CAD build for the part. Positions are in the model's coordinates, mm. Give positions to 0.01 mm unless a question says otherwise; leave off trailing zeros. Write each loop counter-clockwise with the first axis right and the second up, starting at its lowest first coordinate (ties: lowest second). Pieces come first, ordered by that corner, then holes. Notation, with made-up numbers: (-7.75, 39.25) -> (34.25, 39.25) arc R16 cw to (34.25, 65.25) -> close; hole circle Ø7 at (21.25, 83.25). An arc over 180 degrees is marked (long way). Answer in a Markdown table with one row per item. Add a question column.
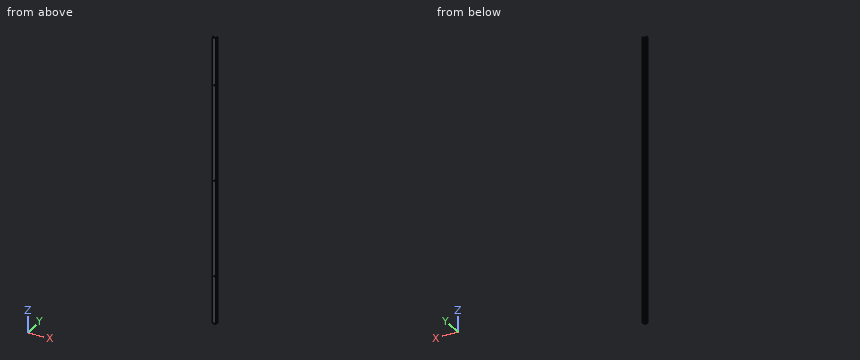
```python
from build123d import *

# Parameters (mm, degrees)
EXTRUDE_THIN1_DEPTH = 2997
SKETCH2_R           = 3.25
CUT_EXTRUDE1_DEPTH  = 2998.203367213
LPATTERN1_COUNT     = 3
LPATTERN1_PITCH     = 1000


with BuildPart() as part:
    # Sketch1 → Extrude-Thin1 (new body)
    with BuildSketch(Plane.XY):
        with BuildLine():
            Line((11.267326733, 18.158415842), (11.267326733, -6.841584158))
            ThreePointArc((11.267326733, -6.841584158), (10.388647076, -8.962904502), (8.267326733, -9.841584158))
            Line((8.267326733, -9.841584158), (-19.732673267, -9.841584158))
            ThreePointArc((-19.732673267, -9.841584158), (-21.853993611, -8.962904502), (-22.732673267, -6.841584158))
            Line((-22.732673267, -6.841584158), (-22.732673267, 18.158415842))
            Line((-22.732673267, 18.158415842), (-21.232673267, 18.158415842))
            Line((-21.232673267, 18.158415842), (-21.232673267, -6.841584158))
            ThreePointArc((-21.232673267, -6.841584158), (-20.793333439, -7.90224433), (-19.732673267, -8.341584158))
            Line((-19.732673267, -8.341584158), (8.267326733, -8.341584158))
            ThreePointArc((8.267326733, -8.341584158), (9.327986904, -7.90224433), (9.767326733, -6.841584158))
            Line((9.767326733, -6.841584158), (9.767326733, 18.158415842))
            Line((9.767326733, 18.158415842), (11.267326733, 18.158415842))
        make_face()
    extrude(amount=EXTRUDE_THIN1_DEPTH)

    # Sketch2 → Cut-Extrude1 (cut, through all)
    with BuildSketch(Plane(origin=(0, -8.341584158, 0), x_dir=(1, 0, 0), z_dir=(0, 1, 0))):
        with Locations(Location((-5.732673267, -2498.5, 0), (0, 0, 180))):
            Circle(SKETCH2_R)
    cut_extrude1 = extrude(amount=-CUT_EXTRUDE1_DEPTH, mode=Mode.SUBTRACT)

    # LPattern1: Cut-Extrude1 ×3
    with Locations(*[(0, 0, -i * LPATTERN1_PITCH) for i in range(1, LPATTERN1_COUNT)]):
        add(cut_extrude1, mode=Mode.SUBTRACT)


solid = part.part
```
Item 1: Slice it at B-B, the plane z = 330.5. List the corners of the cut face in (x, y), then the cut area to 3 significant figures.
Item 2: Drop a flat-ended pin along its axis: pin 1 Ø7.5 at (x, z) = (-5.73, 498.5) entering from +Y. Give the stop position or say it passes through.
Item 3: Probe L1, parallel to X at y = -9.2, z = 498.5; L2, parallel to X at y = -2, z = 468; L3, parallel to Y at x = -18, z = 741. List the from-to ranges inside material, lowest first. Write a range as from..to.
Item 4: Slice it at A-A, the plane y = 12.25. List the corners of the cut face in (x, z), then the cut area to 3 significant figures.
Answer key:
| question | item | result |
|---|---|---|
| 1 | outline | (-22.73, -6.84) arc R3 ccw to (-19.73, -9.84) -> (8.27, -9.84) arc R3 ccw to (11.27, -6.84) -> (11.27, 18.16) -> (9.77, 18.16) -> (9.77, -6.84) arc R1.5 cw to (8.27, -8.34) -> (-19.73, -8.34) arc R1.5 cw to (-21.23, -6.84) -> (-21.23, 18.16) -> (-22.73, 18.16) -> close |
| 1 | area | 128 mm² |
| 2 | pin 1 | stops at y = -8.34 |
| 3 | L1 | x = -21.59..-8.98, -2.48..10.12 |
| 3 | L2 | x = -22.73..-21.23, 9.77..11.27 |
| 3 | L3 | y = -9.84..-8.34 |
| 4 | outline | (-22.73, 0) -> (-21.23, 0) -> (-21.23, 2997) -> (-22.73, 2997) -> close; (9.77, 0) -> (11.27, 0) -> (11.27, 2997) -> (9.77, 2997) -> close |
| 4 | area | 8,990 mm² |
